```python
from build123d import *

# Parameters (mm, degrees)
ESBO_O1_R                = 2
ESBO_O1_R_2              = 1
RESSALTO_EXTRUS_O1_DEPTH = 4
ESBO_O2_R                = 2
RESSALTO_EXTRUS_O2_DEPTH = 2


with BuildPart() as part:
    # Esboço1 → Ressalto-extrusão1 (new body)
    with BuildSketch(Plane(origin=(0, 0, 0), x_dir=(1, 0, 0), z_dir=(0, 1, 0))):
        with Locations(Location((0, 0, 0), (0, 0, 270))):
            Circle(ESBO_O1_R)
        with Locations(Location((0, 0, 0), (0, 0, 270))):
            Circle(ESBO_O1_R_2, mode=Mode.SUBTRACT)
    extrude(amount=RESSALTO_EXTRUS_O1_DEPTH)

    # Esboço2 → Ressalto-extrusão2 (add)
    with BuildSketch(Plane(origin=(0, 4, 0), x_dir=(1, 0, 0), z_dir=(0, 1, 0))):
        with Locations(Location((0, 0, 0), (0, 0, 60))):
            Circle(ESBO_O2_R)
        Polygon((10, 17.320508076), (0, 0), (-10, 17.320508076), align=None)
        Polygon((-10, -17.320508076), (10, -17.320508076), (0, 0), align=None)
    extrude(amount=RESSALTO_EXTRUS_O2_DEPTH)


solid = part.part
```
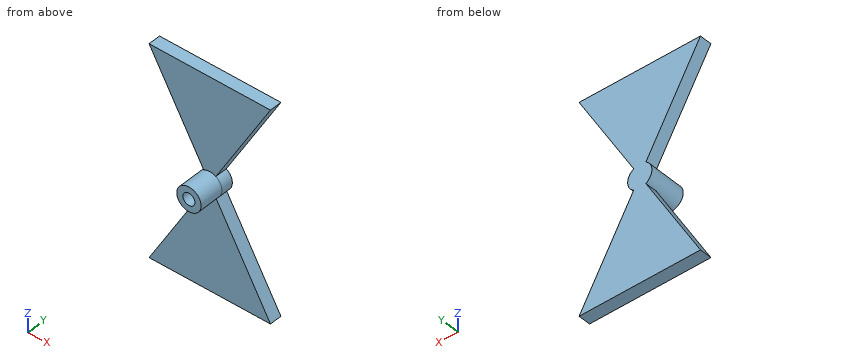
For this review, take the finished solid that the model builds, in its own axes (mm). Give positions to 0.01 mm unless a question says otherwise; leave off trailing zeros. Write each loop counter-clockwise with the first axis right and the second up, starting at its lowest first coordinate (ties: lowest second). Pieces come first, ordered by that corner, then holes. Notation, with made-up numbers: M 62.5,-11 L 108.5,-11 A17 ccw 108.5,3 Z; hole C 2.25,11 d6. An arc over 180 degrees is marked long. Answer as a JSON object with one key per item and string values. Group by question number.
Item 1: Consider section A-A on z = 0. Write out the cut boundary in (x, y).
Item 2: For probe 1 along X at (y, z) = (1.65, 0); probe 2 along X at (y, z) = (0.65, -0.5); probe 3 along Y at (x, z) = (3, 11), list the stretches that pass through material, from the lowest coordinate up. Write a range as [from, to].
Item 3: Consider section C-C on x = 4. Write out the cut boundary in (y, z), plus the area to 3 significant figures.
Item 4: Consider section D-D on y = 2.9. Write out the cut boundary in (x, z).
Item 5: For pin 1 Ø3 at (y, z) = (5, -12.5) entering from -X; pin 2 Ø5 at (x, z) = (-7, 7.5) entering from +Y; pin 3 Ø2 at (y, z) = (4, 0.5) entering from -X; pin 4 Ø1 at (y, z) = (3, -10) entering from -X, all flat-tipped, find the tip position at first contact; note any pin that passes through.
Item 6: Consider section B-B on x = 0. Write out the cut boundary in (y, z), plus the area to 3 significant figures.
Check result:
{
 "1": {"outline": "M -2,0 L -1,0 L -1,4 L 1,4 L 1,0 L 2,0 L 2,6 L -2,6 Z"},
 "2": {"probe 1": "x = [-2, -1], [1, 2]", "probe 2": "x = [-1.94, -0.87], [0.87, 1.94]", "probe 3": "y = [4, 6]"},
 "3": {"outline": "M 4,-17.32 L 6,-17.32 L 6,-6.93 L 4,-6.93 Z; M 4,6.93 L 6,6.93 L 6,17.32 L 4,17.32 Z", "area": "41.6 mm^2"},
 "4": {"outline": "C 0,0 d4; hole C 0,0 d2"},
 "5": {"pin 1": "stops at x = -8.08", "pin 2": "stops at y = 6", "pin 3": "stops at x = -2", "pin 4": "passes through"},
 "6": {"outline": "M 0,-2 L 4,-2 L 4,-17.32 L 6,-17.32 L 6,17.32 L 4,17.32 L 4,2 L 0,2 L 0,1 L 4,1 L 4,-1 L 0,-1 Z", "area": "77.3 mm^2"}
}
